from build123d import *

# Parameters (mm, degrees)
PER_AGE1_D = 6.6


with BuildPart() as part:
    # Esquisse1 → Base-Révolution (revolve)
    with BuildSketch(Plane.XY, mode=Mode.PRIVATE) as base_r_volution_sk:
        Polygon((0, 52.5), (0, 75), (15, 75), (15, 60), (5, 60), (5, 52.5), align=None)
    revolve(base_r_volution_sk.sketch.rotate(Axis((-16.708877928, 0, 0), (1, 0, 0)), 90), axis=Axis((-16.708877928, 0, 0), (1, 0, 0)))

    # Perçage1 (through all)
    with Locations(Plane.ZY):
        with Locations((0, 67.5), (67.5, 0), (0, -67.5), (-67.5, 0)):
            Hole(PER_AGE1_D / 2)


solid = part.part
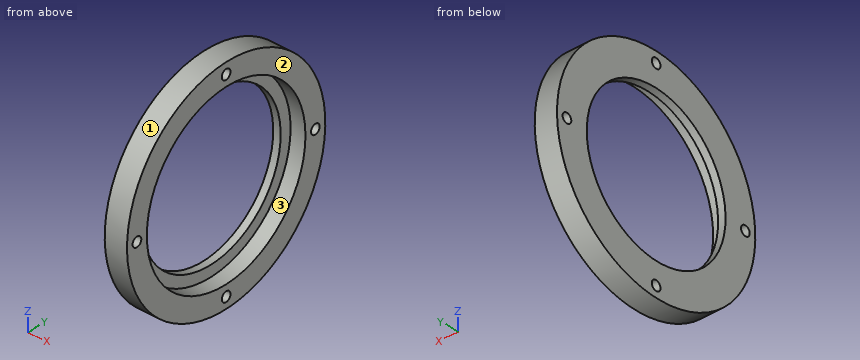
Geometry: final body of the model. Coordinates: model frame, mm. Face numbers are marked on the shaded views. Coordinates: 2 decimals unless noted, no trailing zeros. Order: outer loops, then holes, each group sorted by start corner. A loop starts at its lowest first (then second) coordinate and runs counter-clockwise, first axis right, second up.
1) Section B-B (y = -39.5). Return loops of the section in (x, z), then the cut area to 3 significant figures.
Result sheet:
outline: (0, -63.76) - (15, -63.76) - (15, -45.16) - (5, -45.16) - (5, -34.58) - (0, -34.58) - close; (0, 34.58) - (5, 34.58) - (5, 45.16) - (15, 45.16) - (15, 63.76) - (0, 63.76) - close
area: 664 mm2
2) Section C-C (x = 11.5). Return loops of the section in (y, z), then the cut area to 3 significant figures.
Result sheet:
outline: circle Ø150 at (0, 0); hole circle Ø6.6 at (-67.5, 0); hole circle Ø120 at (0, 0); hole circle Ø6.6 at (0, -67.5); hole circle Ø6.6 at (0, 67.5); hole circle Ø6.6 at (67.5, 0)
area: 6,220 mm2
3) Ray query, probe 1 along Y at (x, z) = (3.2, 0); probe 2 along Y at (x, z) = (10.5, 0); probe 3 along Z at (x, y) = (2.5, -2.5). Return the intervals inside material, ascending.
Result sheet:
probe 1: y = -75 to -70.8, -64.2 to -52.5, 52.5 to 64.2, 70.8 to 75
probe 2: y = -75 to -70.8, -64.2 to -60, 60 to 64.2, 70.8 to 75
probe 3: z = -74.96 to -69.65, -65.35 to -52.44, 52.44 to 65.35, 69.65 to 74.96
4) Draft query along Y for the marked faces 1, 2 and 3. Return one class per face: released by +Y, released by -Y, zero draft, split by the parting line, or undercut.
Result sheet:
face 1: split by the parting line
face 2: zero draft
face 3: undercut
5) Section D-D (z = -19). Return loops of the section in (x, y).
Result sheet:
outline: (0, -72.55) - (15, -72.55) - (15, -56.91) - (5, -56.91) - (5, -48.94) - (0, -48.94) - close; (0, 48.94) - (5, 48.94) - (5, 56.91) - (15, 56.91) - (15, 72.55) - (0, 72.55) - close
6) First-contact query: P1, Ø6, axis at y = 0, z = -67.5, coming from the +X side; P2, Ø6, axis at x = 13.5, z = 57, coming from the -Y side; P3, Ø1.5, axis at x = 6.5, y = -51.5, coming from the +Z side; P4, Ø12, axis at y = 46, z = 24.5, coming from the +X side. Flat tips, straight axial feed; report the tip coordinate or a pass-through.
Result sheet:
P1: passes through
P2: stops at y = -52.05
P3: stops at z = 55.22
P4: stops at x = 5
7) Section A-A (z = 0). Return loops of the section in (x, y), then the cut area to 3 significant figures.
Result sheet:
outline: (0, -75) - (15, -75) - (15, -70.8) - (0, -70.8) - close; (0, -64.2) - (15, -64.2) - (15, -60) - (5, -60) - (5, -52.5) - (0, -52.5) - close; (0, 52.5) - (5, 52.5) - (5, 60) - (15, 60) - (15, 64.2) - (0, 64.2) - close; (0, 70.8) - (15, 70.8) - (15, 75) - (0, 75) - close
area: 327 mm2
